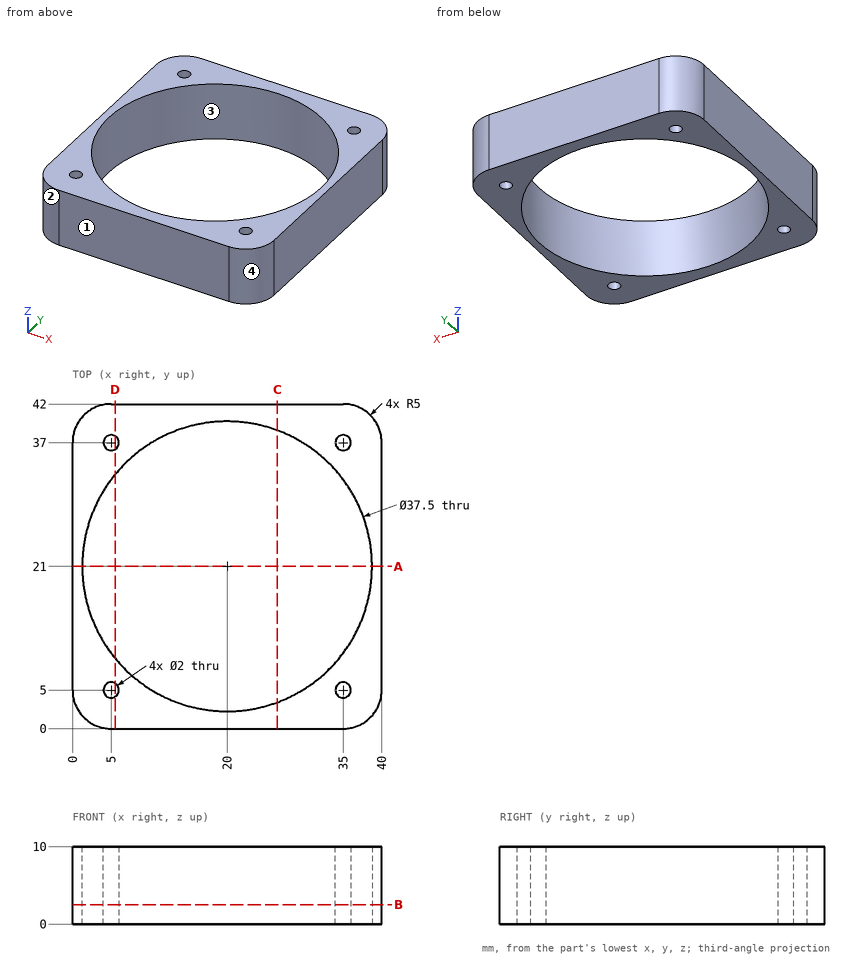
The figure shows three views and two pictorial views of one solid part (mm, origin at its lowest corner). Answer the questions. Round coordinates to 2 decimals unless told otherwise and drop trailing zeros. Order: outer loops, then holes, each group sorted by start corner. A loop starts at its lowest first (then second) coordinate and runs counter-clockwise, first axis right, second up.
Q1. A cutting plane is placed at C-C, the plane x = 26.5. Determine the outline of the cut face in (y, z).
Solution:
outline: (0, 0) - (3.41, 0) - (3.41, 10) - (0, 10) - close; (38.59, 0) - (42, 0) - (42, 10) - (38.59, 10) - close
Q2. A cutting plane is placed at A-A, the plane y = 21. Determine the outline of the cut face in (x, z), then the cut area to 3 significant figures.
Solution:
outline: (0, 0) - (1.25, 0) - (1.25, 10) - (0, 10) - close; (38.75, 0) - (40, 0) - (40, 10) - (38.75, 10) - close
area: 25.0 mm2
Q3. The mould has two halves that part along X. Classify the marked faces 1, 2, 3 and 4: pulls with the +X half, pulls with the -X half, needs draft (parallel to the pull), parting line crosses it, or undercut.
Solution:
face 1: needs draft
face 2: pulls with the -X half
face 3: undercut
face 4: pulls with the +X half
Q4. A cutting plane is placed at D-D, the plane x = 5.5. Determine the outline of the cut face in (y, z).
Solution:
outline: (0, 0) - (4.13, 0) - (4.13, 10) - (0, 10) - close; (5.87, 0) - (9.11, 0) - (9.11, 10) - (5.87, 10) - close; (32.89, 0) - (36.13, 0) - (36.13, 10) - (32.89, 10) - close; (37.87, 0) - (42, 0) - (42, 10) - (37.87, 10) - close
Q5. A cutting plane is placed at B-B, the plane z = 2.5. Determine the outline of the cut face in (x, y), then the cut area to 3 significant figures.
Solution:
outline: (0, 5) arc R5 ccw to (5, 0) - (35, 0) arc R5 ccw to (40, 5) - (40, 37) arc R5 ccw to (35, 42) - (5, 42) arc R5 ccw to (0, 37) - close; hole circle Ø37.5 at (20, 21); hole circle Ø2 at (5, 5); hole circle Ø2 at (5, 37); hole circle Ø2 at (35, 5); hole circle Ø2 at (35, 37)
area: 542 mm2
Q6. Find the intervals of material crossed by line 1 along Y through (x, z) = (20, 7.25); line 2 along Y through (x, z) = (5, 8); line 3 along Y through (x, z) = (27.5, 2.25), in increasing order.
Solution:
line 1: y = 0 to 2.25, 39.75 to 42
line 2: y = 0 to 4, 6 to 9.75, 32.25 to 36, 38 to 42
line 3: y = 0 to 3.82, 38.18 to 42
